The model under review builds one solid part; all positions refer to its coordinate system, in mm. Face numbers are marked on the shaded views. Coordinates: 2 decimals unless noted, no trailing zeros. Order: outer loops, then holes, each group sorted by start corner. A loop starts at its lowest first (then second) coordinate and runs counter-clockwise, first axis right, second up. Notation, with made-up numbers: M 53.25,26.25 L 111.25,26.25 A6 ccw 111.25,30.25 Z; hole C 85,-21.5 d1. An arc over 180 degrees is marked long. Answer in a Markdown table with one row per item.
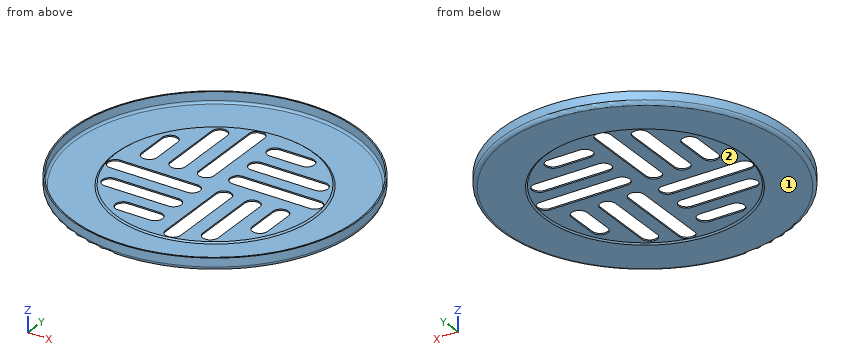
from build123d import *

# Parameters (mm, degrees)
F3_DEPTH = 4.896274


with BuildPart() as f1:
    # F0 (on Front) → F1 (revolve)
    with BuildSketch(Plane.XZ):
        with BuildLine():
            Line((-65, 1), (-65, 4.895274))
            Line((-65, 4.895274), (-65.6, 4.895274))
            Line((-65.6, 4.895274), (-65.6, 1))
            ThreePointArc((-65.6, 1), (-65.131371, -0.131371), (-64, -0.6))
            Line((-64, -0.6), (-45.582217, -0.6))
            Line((-45.582217, -0.6), (-44.797003, 0))
            Line((-44.797003, 0), (0, 0))
            Line((0, 0), (0, 0.6))
            Line((0, 0.6), (-45, 0.6))
            Line((-45, 0.6), (-45.785214, 0))
            Line((-45.785214, 0), (-64, 0))
            ThreePointArc((-64, 0), (-64.707107, 0.292893), (-65, 1))
        make_face()
    revolve(axis=Axis((0, 0, 2.485013), (0, 0, -1)))

    # F2 (on Top) → F3 (cut, through all)
    with BuildSketch(Plane.XY):
        with BuildLine():
            Line((-5.467376, -4), (-40.467376, -4))
            ThreePointArc((-40.467376, -4), (-44.034095, -7.466402), (-40.533936, -11))
            Line((-40.533936, -11), (-5.467376, -11))
            ThreePointArc((-5.467376, -11), (-1.967376, -7.5), (-5.467376, -4))
        make_face()
        with BuildLine():
            Line((-5.467376, -17), (-34.467376, -17))
            ThreePointArc((-34.467376, -17), (-37.967376, -20.5), (-34.467376, -24))
            Line((-34.467376, -24), (-5.467376, -24))
            ThreePointArc((-5.467376, -24), (-1.967376, -20.5), (-5.467376, -17))
        make_face()
        with BuildLine():
            Line((-5.467376, -30), (-19.874607, -30))
            ThreePointArc((-19.874607, -30), (-23.374607, -33.5), (-19.874607, -37))
            Line((-19.874607, -37), (-5.467376, -37))
            ThreePointArc((-5.467376, -37), (-1.967376, -33.5), (-5.467376, -30))
        make_face()
        with BuildLine():
            ThreePointArc((-30, 19.874607), (-33.5, 23.374607), (-37, 19.874607))
            Line((-37, 19.874607), (-37, 5.467376))
            ThreePointArc((-37, 5.467376), (-33.5, 1.967376), (-30, 5.467376))
            Line((-30, 5.467376), (-30, 19.874607))
        make_face()
        with BuildLine():
            ThreePointArc((-17, 34.467376), (-20.5, 37.967376), (-24, 34.467376))
            Line((-24, 34.467376), (-24, 5.467376))
            ThreePointArc((-24, 5.467376), (-20.5, 1.967376), (-17, 5.467376))
            Line((-17, 5.467376), (-17, 34.467376))
        make_face()
        with BuildLine():
            ThreePointArc((-4, 40.467376), (-7.466402, 44.034095), (-11, 40.533936))
            Line((-11, 40.533936), (-11, 5.467376))
            ThreePointArc((-11, 5.467376), (-7.5, 1.967376), (-4, 5.467376))
            Line((-4, 5.467376), (-4, 40.467376))
        make_face()
        with BuildLine():
            Line((17, -5.467376), (17, -34.467376))
            ThreePointArc((17, -34.467376), (20.5, -37.967376), (24, -34.467376))
            Line((24, -34.467376), (24, -5.467376))
            ThreePointArc((24, -5.467376), (20.5, -1.967376), (17, -5.467376))
        make_face()
        with BuildLine():
            Line((4, -5.467376), (4, -40.467376))
            ThreePointArc((4, -40.467376), (7.466402, -44.034095), (11, -40.533936))
            Line((11, -40.533936), (11, -5.467376))
            ThreePointArc((11, -5.467376), (7.5, -1.967376), (4, -5.467376))
        make_face()
        with BuildLine():
            Line((30, -5.467376), (30, -19.874607))
            ThreePointArc((30, -19.874607), (33.5, -23.374607), (37, -19.874607))
            Line((37, -19.874607), (37, -5.467376))
            ThreePointArc((37, -5.467376), (33.5, -1.967376), (30, -5.467376))
        make_face()
        with BuildLine():
            Line((5.467376, 4), (40.467376, 4))
            ThreePointArc((40.467376, 4), (44.034095, 7.466402), (40.533936, 11))
            Line((40.533936, 11), (5.467376, 11))
            ThreePointArc((5.467376, 11), (1.967376, 7.5), (5.467376, 4))
        make_face()
        with BuildLine():
            Line((5.467376, 17), (34.467376, 17))
            ThreePointArc((34.467376, 17), (37.967376, 20.5), (34.467376, 24))
            Line((34.467376, 24), (5.467376, 24))
            ThreePointArc((5.467376, 24), (1.967376, 20.5), (5.467376, 17))
        make_face()
        with BuildLine():
            Line((5.467376, 30), (19.874607, 30))
            ThreePointArc((19.874607, 30), (23.374607, 33.5), (19.874607, 37))
            Line((19.874607, 37), (5.467376, 37))
            ThreePointArc((5.467376, 37), (1.967376, 33.5), (5.467376, 30))
        make_face()
    extrude(amount=F3_DEPTH, mode=Mode.SUBTRACT)


solid = f1.part
(1) Take a section at B-B (z = 3.3). Write out the cut boundary in (x, y), then the cut area to 3 significant figures.
Report:
| item | result |
|---|---|
| outline | C 0,0 d131.2; hole C 0,0 d130 |
| area | 246 mm^2 |
(2) Take a section at A-A (x = 0). Write out the cut boundary in (y, z), then the cut area to 3 significant figures.
Report:
| item | result |
|---|---|
| outline | M -65.6,1 A1.6 ccw -64,-0.6 L -45.58,-0.6 L -44.8,0 L 44.8,0 L 45.58,-0.6 L 64,-0.6 A1.6 ccw 65.6,1 L 65.6,4.9 L 65,4.9 L 65,1 A1 cw 64,0 L 45.79,0 L 45,0.6 L -45,0.6 L -45.79,0 L -64,0 A1 cw -65,1 L -65,4.9 L -65.6,4.9 Z |
| area | 84.2 mm^2 |
(3) The part is to be moulded in two halves that separate along Y. For the marked faces 1 and 2, say which applies: +Y half, -Y half, draft (parallel to the pull), parting line (faces both ways), or undercut.
Report:
| item | result |
|---|---|
| face 1 | draft |
| face 2 | undercut |
(4) To check wall thickness, follow line 1 (Y direction, x = 0, z = 2.8); line 2 (Z direction, x = 49, y = 19); line 3 (X direction, y = -35, z = 0.4). State the ranges of each line that lie inside material, in increasing order. Write a range as [from, to].
Report:
| item | result |
|---|---|
| line 1 | [-65.6, -65], [65, 65.6] |
| line 2 | [-0.6, 0] |
| line 3 | [-55.34, -54.53], [-28.7, -23.04], [-2.31, 4], [11, 17.04], [23.96, 28.7], [54.53, 55.34] |
(5) Take a section at C-C (x = 25.5). State how many separate pieces and enclosed holes the cut face has, then the cut area to 3 significant figures.
Report:
| item | result |
|---|---|
| separate pieces | 3 |
| enclosed holes | 0 |
| area | 70.1 mm^2 |
(6) Insertion check: P1, Ø0.5, axis at y = 13.5, z = 0.5, coming from the +X side; P2, Ø0.7, axis at x = -15.5, z = 0.5, coming from the +Y side; P3, Ø3, axis at x = -29, z = 3, coming from the -Y side. Each pin has a flat end and moves straight along its axis. Give the tip position at first contact, or say it passes through.
Report:
| item | result |
|---|---|
| P1 | x = 64.2 |
| P2 | y = 63.78 |
| P3 | y = -59.56 |
